Here's how the part is built. I have some questions about the finished solid (model axes, mm). Round coordinates to 2 decimals unless told otherwise and drop trailing zeros. Order: outer loops, then holes, each group sorted by start corner. A loop starts at its lowest first (then second) coordinate and runs counter-clockwise, first axis right, second up. Notation, with made-up numbers: M 37,32 L 73,32 A19 cw 73,40 Z; hole C -27,24.5 d3. An arc over 180 degrees is marked long. Write item = value, one per line. Start each with the question number.
Item 1: I want a section at B-B, the plane x = 125.5. List the corners of the cut face in (y, z) for me, plus the area to 3 significant figures.
Item 2: I'm going to push flat-ended pins straight in: P1, Ø6.5, axis at x = 103.87, z = 14.1, coming from the +Y side; P2, Ø5, axis at x = 91.5, y = -116.5, coming from the +Z side; P3, Ø4, axis at x = 145.5, z = 13, coming from the +Y side. Where does each tip first touch, or does it pass through?
Item 3: Please list where these lines run through material, in increasing order: L1, parallel to Z at x = 187.41, y = -118.55; L2, parallel to Z at x = 188.21, y = -112.95; L3, parallel to Z at x = 74.12, y = -115.65.
Item 4: I want a section at A-A, the plane z = 49. List the corners of the cut face in (x, y) for me.
Item 5: I want a section at C-C, the plane x = 74.12. List the corners of the cut face in (y, z) for me.
```python
from build123d import *

# Parameters (mm, degrees)
PAD017_DEPTH    = 1
PAD018_DEPTH    = 2
SKETCH041_R     = 3.5
PAD019_DEPTH    = 3.3
SKETCH042_R     = 2.55
POCKET018_DEPTH = 4.3
SKETCH043_R     = 2.8
PAD020_DEPTH    = 1.5
SKETCH044_R     = 2.1
POCKET019_DEPTH = 3
SKETCH045_R     = 3.5
PAD021_DEPTH    = 5.8
SKETCH046_R     = 2.55
POCKET020_DEPTH = 3.8
SKETCH047_R     = 2.5
POCKET021_DEPTH = 1.7
POCKET025_DEPTH = 2


with BuildPart() as part:
    # Sketch038 → Pad017 (new body)
    with BuildSketch(Plane.XZ):
        with BuildLine():
            ThreePointArc((6, 16), (8.928932, 8.928932), (16, 6))
            Line((16, 6), (185.51, 6))
            ThreePointArc((185.51, 6), (192.581068, 8.928932), (195.51, 16))
            Line((195.51, 16), (195.51, 107.04))
            ThreePointArc((195.51, 107.04), (192.581068, 114.111068), (185.51, 117.04))
            Line((185.51, 117.04), (96.718237, 117.04))
            ThreePointArc((96.718237, 117.04), (95.677689, 117.177713), (94.70879, 117.58137))
            Line((94.70879, 117.58137), (67.290497, 133.511257))
            ThreePointArc((67.290497, 133.511257), (65.837149, 134.116742), (64.276328, 134.323311))
            Line((64.276328, 134.323311), (41.441667, 134.323311))
            ThreePointArc((41.441667, 134.323311), (36.445319, 132.985672), (32.785632, 129.330611))
            Line((32.785632, 129.330611), (9.11531, 88.412125))
            ThreePointArc((9.11531, 88.412125), (6.792371, 82.814067), (6, 76.805203))
            Line((6, 76.805203), (6, 16))
        make_face()
    extrude(amount=PAD017_DEPTH)

    # Sketch040 (on Face15 of Pad017) → Pad018 (join)
    with BuildSketch(Plane(origin=(0, 0, 0), x_dir=(1, 0, 0), z_dir=(0, 1, 0))):
        with BuildLine():
            Line((16.1, -9.1), (185.41, -9.1))
            ThreePointArc((192.41, -16.1), (190.359747, -11.150253), (185.41, -9.1))
            Line((192.41, -16.1), (192.41, -106.94))
            ThreePointArc((185.41, -113.94), (190.359747, -111.889747), (192.41, -106.94))
            Line((185.41, -113.94), (95.883059, -113.94))
            ThreePointArc((95.883059, -113.94), (94.842511, -114.077713), (93.873612, -114.48137))
            Line((93.873612, -114.48137), (66.455319, -130.411257))
            ThreePointArc((63.44115, -131.223311), (65.001971, -131.016742), (66.455319, -130.411257))
            Line((63.44115, -131.223311), (41.499346, -131.223311))
            ThreePointArc((35.440122, -127.728421), (38.001902, -130.286964), (41.499346, -131.223311))
            Line((35.440122, -127.728421), (12.21531, -87.580081))
            ThreePointArc((9.1, -75.97316), (9.892371, -81.982024), (12.21531, -87.580081))
            Line((9.1, -75.97316), (9.1, -16.1))
            ThreePointArc((16.1, -9.1), (11.150253, -11.150253), (9.1, -16.1))
        make_face()
    extrude(amount=PAD018_DEPTH)

    # Sketch041 (on Face31 of Pad018) → Pad019 (join)
    with BuildSketch(Plane(origin=(0, 2, 0), x_dir=(1, 0, 0), z_dir=(0, 1, 0))):
        with Locations((145.11, -12.99)):
            Circle(SKETCH041_R)
        with Locations((64.452126, -127.45504)):
            Circle(SKETCH041_R)
        with Locations((14.14, -13.51)):
            Circle(SKETCH041_R)
        with Locations((19.14, -90.503884)):
            Circle(SKETCH041_R)
        with Locations((105.9, -108.54)):
            Circle(SKETCH041_R)
        with Locations((74.12, -12.75)):
            Circle(SKETCH041_R)
    extrude(amount=PAD019_DEPTH)

    # Sketch042 (on Face38 of Pad019) → Pocket018 (cut)
    with BuildSketch(Plane(origin=(0, 5.3, 0), x_dir=(1, 0, 0), z_dir=(0, 1, 0))):
        with Locations((145.11, -12.99)):
            Circle(SKETCH042_R)
        with Locations((19.14, -90.503884)):
            Circle(SKETCH042_R)
        with Locations((64.452126, -127.45504)):
            Circle(SKETCH042_R)
        with Locations((105.9, -108.54)):
            Circle(SKETCH042_R)
        with Locations((14.14, -13.51)):
            Circle(SKETCH042_R)
        with Locations((74.12, -12.75)):
            Circle(SKETCH042_R)
    extrude(amount=-POCKET018_DEPTH, mode=Mode.SUBTRACT)

    # Sketch043 (on Face31 of Pocket018) → Pad020 (join)
    with BuildSketch(Plane(origin=(0, 2, 0), x_dir=(1, 0, 0), z_dir=(0, 1, 0))):
        with Locations((185.580566, -111.078545)):
            Circle(SKETCH043_R)
    extrude(amount=PAD020_DEPTH)

    # Sketch044 (on Face45 of Pad020) → Pocket019 (cut)
    with BuildSketch(Plane(origin=(0, 3.5, 0), x_dir=(1, 0, 0), z_dir=(0, 1, 0))):
        with Locations((185.580566, -111.078545)):
            Circle(SKETCH044_R)
    extrude(amount=-POCKET019_DEPTH, mode=Mode.SUBTRACT)

    # Sketch045 (on Face31 of Pocket019) → Pad021 (join)
    with BuildSketch(Plane(origin=(0, 2, 0), x_dir=(1, 0, 0), z_dir=(0, 1, 0))):
        with Locations((188.21, -14.18)):
            Circle(SKETCH045_R)
    extrude(amount=PAD021_DEPTH)

    # Sketch046 (on Face45 of Pad021) → Pocket020 (cut)
    with BuildSketch(Plane(origin=(0, 7.8, 0), x_dir=(1, 0, 0), z_dir=(0, 1, 0))):
        with Locations((188.21, -14.18)):
            Circle(SKETCH046_R)
    extrude(amount=-POCKET020_DEPTH, mode=Mode.SUBTRACT)

    # Sketch047 (on Face5 of Pocket020) → Pocket021 (cut)
    with BuildSketch(Plane.XZ.offset(1)):
        with Locations((187.41, 103.94)):
            Circle(SKETCH047_R)
        with Locations((40.34577, 126.223311)):
            Circle(SKETCH047_R)
        with Locations((14.1, 77.580081)):
            Circle(SKETCH047_R)
        with Locations((103.873612, 14.1)):
            Circle(SKETCH047_R)
        with Locations((187.41, 19.1)):
            Circle(SKETCH047_R)
        with Locations((120.883059, 108.94)):
            Circle(SKETCH047_R)
        with Locations((19.1, 14.1)):
            Circle(SKETCH047_R)
    extrude(amount=-POCKET021_DEPTH, mode=Mode.SUBTRACT)

    # Sketch056 (on Face38 of Pocket021) → Pocket025 (cut)
    with BuildSketch(Plane(origin=(0, 2, 0), x_dir=(1, 0, 0), z_dir=(0, 1, 0))):
        Polygon((146.906174, -8.786863), (146.906174, -9.81445), (150.102356, -9.81445), (150.102356, -15.780038), (161.659576, -15.780038), (161.659576, -9.891122), (164.762894, -9.891122), (164.762894, -8.786863), align=None)
    extrude(amount=-POCKET025_DEPTH, mode=Mode.SUBTRACT)


with BuildPart() as part_1:
    # Body004 placement: moved
    add(part.part.moved(Location((0, -118.5, 0))))


solid = part_1.part
```
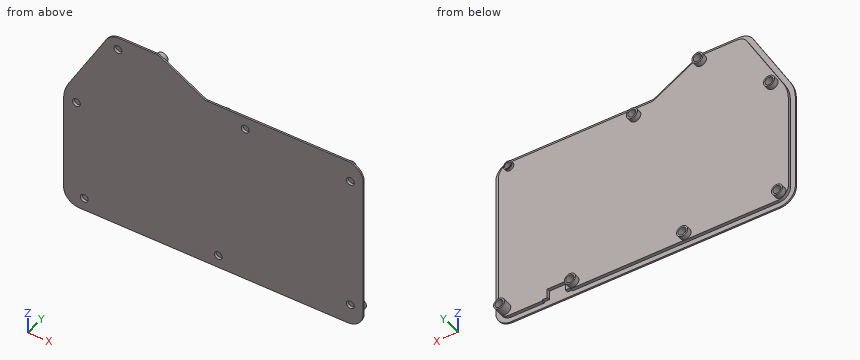
Filled in:
q1.outline = M -119.5,6 L -118.5,6 L -118.5,9.1 L -116.5,9.1 L -116.5,113.94 L -118.5,113.94 L -118.5,117.04 L -119.5,117.04 Z
q1.area = 321 mm^2
q2.P1 = -116.5
q2.P2 = 120.32
q2.P3 = -117.5
q3.L1 = 6.18 to 16.6, 21.6 to 101.44, 106.44 to 116.86
q3.L2 = 10.68 to 11.63, 16.73 to 17.68
q3.L3 = 9.25 to 10.2, 15.3 to 16.25
q4.outline = M 6,-119.5 L 195.51,-119.5 L 195.51,-118.5 L 192.41,-118.5 L 192.41,-116.5 L 9.1,-116.5 L 9.1,-118.5 L 6,-118.5 Z
q5.outline = M -119.5,6 L -118.5,6 L -118.5,9.1 L -116.5,9.1 L -116.5,9.25 L -113.2,9.25 L -113.2,10.2 L -117.5,10.2 L -117.5,15.3 L -113.2,15.3 L -113.2,16.25 L -116.5,16.25 L -116.5,125.96 L -118.5,125.96 L -118.5,129.54 L -119.5,129.54 Z
